Could you check a few things on this model? Use its own coordinates, in mm. A direction names the side the tool comes from. Round coordinates to 2 decimals unless told otherwise and drop trailing zeros. Loops run counter-clockwise (first coordinate to the right, second up) from the corner with the lowest first, then second, coordinate; pieces in that order, holes last. Notation, with made-up numbers: M 38.5,36.5 L 44.5,36.5 A9 cw 44.5,47.5 Z; hole C 5.5,-34 d5. An arc over 180 degrees is marked long. Return JSON: item names as keys, results as strings. Group by question number.
Autodesk Fusion 360 part; units mm, degrees
sketch "Sketch1" plane through (0, 0, 0) normal (0, 0, 1) x (1, 0, 0)
  line L0 (0, 0) -> (10.75, 0)
  line L1 (10.75, 0) -> (10.75, 10.75)
  line L2 (10.75, 10.75) -> (0, 10.75)
  line L3 (0, 10.75) -> (0, 0)
  dimension "d1" = 10.75
  dimension "d2" = 10.75
extrude "Extrude1" add sketch "Sketch1" along normal blind 4
sketch "Sketch2" plane through (0, 0, 4) normal (0, 0, 1) x (-1, 0, 0)
  line L0 (0, -10.75) -> (0, 0)
  line L1 (0, 0) -> (-10.75, 0)
  line L2 (-10.75, 0) -> (-10.75, -10.75)
  line L3 (-10.75, -10.75) -> (0, -10.75)
  circle A0 centre (-5.375, -5.375) radius 4.4
  dimension "d5" = 8.8
extrude "Extrude2" add sketch "Sketch2" along normal blind 14 contours A0
1. I need wall thicknesses on probe 1 along Z at (x, y) = (5.5, 10.25); probe 2 along X at (y, z) = (5.25, 15); probe 3 along X at (y, z) = (2.75, 7.5). Which ranges of each line are inside material? Lowest first, please.
2. On a 3-axis mill with a long thin cutter (end or side, diameter ignored), from which of +Z, -Z, +X, -X, +Y, -Y can I reach the whole of each face in a straight line? I mean faces 1 (the face through (5.948, 9.738, 10.902)), 2 (the face through (5, 10.75, 2)). Say none if no direction works.
3. If we section it at D-D, the plane z = 12.5: Please give me the cut outline in (x, y) (3 decimals), then the cut area to 3 significant figures.
4. If we section it at B-B, the plane x = 0.75: Please give me the cut outline in (y, z), then the cut area to 3 significant figures.
5. I'm going to push flat-ended pins straight in: pin 1 Ø5 at (x, z) = (7.5, 12) entering from -Y (3 decimals); pin 2 Ø4 at (y, z) = (5, 12) entering from -X (3 decimals); pin 3 Ø1.5 at (x, z) = (1.5, 13) entering from +Y. Where does each tip first touch, or does it pass through?
6. If we section it at C-C, the plane y = 1.25: Please give me the cut outline in (x, z).
7. If we section it at A-A, the plane y = 6: Please give me the cut outline in (x, z).
Geometry results:
{
 "1": {"probe 1": "0 to 4", "probe 2": "0.98 to 9.77", "probe 3": "1.84 to 8.91"},
 "2": {"face 1": "+Z", "face 2": "+Z, -Z, +X, -X, +Y"},
 "3": {"outline": "C 5.375,5.375 d8.8", "area": "60.8 mm^2"},
 "4": {"outline": "M 0,0 L 10.75,0 L 10.75,4 L 0,4 Z", "area": "43.0 mm^2"},
 "5": {"pin 1": "y = 0.975", "pin 2": "x = 0.975", "pin 3": "y = 8.47"},
 "6": {"outline": "M 0,0 L 10.75,0 L 10.75,4 L 6.91,4 L 6.91,18 L 3.84,18 L 3.84,4 L 0,4 Z"},
 "7": {"outline": "M 0,0 L 10.75,0 L 10.75,4 L 9.73,4 L 9.73,18 L 1.02,18 L 1.02,4 L 0,4 Z"}
}
